Can you work these out from the model? Positions are in its coordinate system, mm. A direction names the side the tool comes from. Round coordinates to 2 decimals unless told otherwise and drop trailing zeros. Order: outer loops, then holes, each group sorted by start corner. A loop starts at its lowest first (then second) coordinate and runs counter-clockwise, first axis right, second up. Notation, with made-up numbers: M 58.25,7.5 L 115.25,7.5 A7 ccw 115.25,19.5 Z; hole C 44,-19 d2. An arc over 180 degrees is marked long. One line per question, with ' | ' between items.
```python
from build123d import *

# Parameters (mm, degrees)
BOSS_EXTRUDE1_DEPTH = 3
SKETCH2_R           = 2
BOSS_EXTRUDE2_DEPTH = 10
SKETCH3_R           = 1.1
CUT_EXTRUDE1_DEPTH  = 10
SKETCH4_W           = 26.4
SKETCH4_H           = 15.8
SKETCH4_W_2         = 22.4
SKETCH4_H_2         = 11.8
BOSS_EXTRUDE3_DEPTH = 4.3
BOSS_EXTRUDE4_DEPTH = 4.3
SKETCH6_R           = 1.1
CUT_EXTRUDE2_DEPTH  = 20.3
SKETCH7_W           = 16.276669309
SKETCH7_H           = 13.12120508
CUT_EXTRUDE3_DEPTH  = 20.3
BOSS_EXTRUDE5_DEPTH = 3
CUT_EXTRUDE4_START  = -21
SKETCH10_R          = 2
CUT_EXTRUDE4_DEPTH  = 21


with BuildPart() as part:
    # Sketch1 → Boss-Extrude1 (new body)
    with BuildSketch(Plane(origin=(0, 0, 0), x_dir=(1, 0, 0), z_dir=(0, 1, 0))):
        with BuildLine():
            Line((-30.38926404, 6.174917902), (-40.065448474, 32.76001614))
            Line((-40.065448474, 32.76001614), (40.065448474, 32.76001614))
            Line((40.065448474, 32.76001614), (30.38926404, 6.174917902))
            ThreePointArc((30.38926404, 6.174917902), (30.206247108, 3.382619115), (31.552193238, 0.929283279))
            Line((31.552193238, 0.929283279), (33.658129878, -1.17665336))
            ThreePointArc((33.658129878, -1.17665336), (34.741993634, -2.798770105), (35.122595972, -4.712187266))
            Line((35.122595972, -4.712187266), (35.122595972, -23.310725409))
            Line((35.122595972, -23.310725409), (-35.122595972, -23.310725409))
            Line((-35.122595972, -23.310725409), (-35.122595972, -4.712187266))
            ThreePointArc((-35.122595972, -4.712187266), (-34.741993634, -2.798770105), (-33.658129878, -1.17665336))
            Line((-33.658129878, -1.17665336), (-31.552193238, 0.929283279))
            ThreePointArc((-31.552193238, 0.929283279), (-30.206247108, 3.382619115), (-30.38926404, 6.174917902))
        make_face()
    extrude(amount=BOSS_EXTRUDE1_DEPTH)

    # Sketch2 → Boss-Extrude2 (add)
    with BuildSketch(Plane(origin=(0, 3, 0), x_dir=(1, 0, 0), z_dir=(0, 1, 0))):
        with Locations(Location((17.5, 0, 0), (0, 0, 270))):
            Circle(SKETCH2_R)
        with Locations(Location((-17.5, 0, 0), (0, 0, 270))):
            Circle(SKETCH2_R)
    extrude(amount=BOSS_EXTRUDE2_DEPTH)

    # Sketch3 → Cut-Extrude1 (cut)
    with BuildSketch(Plane(origin=(0, 3, 0), x_dir=(1, 0, 0), z_dir=(0, 1, 0))):
        with Locations(Location((-31.300794494, -15.24150981, 0), (0, 0, 270))):
            Circle(SKETCH3_R)
        with Locations(Location((-3.502149082, -14.967077195, 0), (0, 0, 270))):
            Circle(SKETCH3_R)
    extrude(amount=-CUT_EXTRUDE1_DEPTH, mode=Mode.SUBTRACT)

    # Sketch4 → Boss-Extrude3 (add)
    with BuildSketch(Plane.XZ):
        with Locations((-17.401471788, 15.214861671)):
            Rectangle(SKETCH4_W, SKETCH4_H)
        with Locations((-17.401471788, 15.214861671)):
            Rectangle(SKETCH4_W_2, SKETCH4_H_2, mode=Mode.SUBTRACT)
    extrude(amount=BOSS_EXTRUDE3_DEPTH)

    # Sketch5 → Boss-Extrude4 (add)
    with BuildSketch(Plane.XZ):
        Polygon((-30.601471788, 23.114861671), (-30.601471788, 7.314861671), (-33.601471788, 9.046912478), (-33.601471788, 21.382810863), align=None)
        Polygon((-1.201471788, 21.382810863), (-4.201471788, 23.114861671), (-4.201471788, 7.314861671), (-1.201471788, 9.046912478), align=None)
    extrude(amount=BOSS_EXTRUDE4_DEPTH)

    # Sketch6 → Cut-Extrude2 (cut)
    with BuildSketch(Plane(origin=(0, 3, 0), x_dir=(1, 0, 0), z_dir=(0, 1, 0))):
        with Locations(Location((-31.300794494, -15.24150981, 0), (0, 0, 270))):
            Circle(SKETCH6_R)
        with Locations(Location((-3.502149082, -14.967077195, 0), (0, 0, 270))):
            Circle(SKETCH6_R)
    extrude(amount=-CUT_EXTRUDE2_DEPTH, mode=Mode.SUBTRACT)

    # Sketch7 → Cut-Extrude3 (cut)
    with BuildSketch(Plane.XZ):
        with Locations((-13.786077898, 14.682620826)):
            Rectangle(SKETCH7_W, SKETCH7_H)
    extrude(amount=-CUT_EXTRUDE3_DEPTH, mode=Mode.SUBTRACT)

    # Sketch8 → Boss-Extrude5 (add)
    with BuildSketch(Plane(origin=(0, 3, 0), x_dir=(1, 0, 0), z_dir=(0, 1, 0))):
        Polygon((-35.122595972, -23.310725409), (35.122595972, -23.310725409), (25.122595972, -33.310725409), (-25.122595972, -33.310725409), align=None)
    extrude(amount=-BOSS_EXTRUDE5_DEPTH)

    # Sketch10 → Cut-Extrude4 (cut)
    with BuildSketch(Plane(origin=(0, 13, 0), x_dir=(1, 0, 0), z_dir=(0, 1, 0)).offset(CUT_EXTRUDE4_START)):
        with Locations(Location((-17.5, 0, 0), (0, 0, 270))):
            Circle(SKETCH10_R)
        with Locations(Location((17.5, 0, 0), (0, 0, 270))):
            Circle(SKETCH10_R)
    extrude(amount=CUT_EXTRUDE4_DEPTH, mode=Mode.SUBTRACT)


solid = part.part
```
(1) If we section it at C-C on x = 17.5: Please give me the cut outline in (y, z).
Final values:
outline: M 0,-32.76 L 3,-32.76 L 3,-2 L 0,-2 Z; M 0,2 L 3,2 L 3,33.31 L 0,33.31 Z
(2) If we section it at A-A on z = 18: Please give me the cut outline in (x, y).
Final values:
outline: M -35.12,0 L -33.6,0 L -33.6,-4.3 L -28.6,-4.3 L -28.6,0 L -21.92,0 L -21.92,3 L -35.12,3 Z; M -6.2,-4.3 L -1.2,-4.3 L -1.2,0 L 35.12,0 L 35.12,3 L -5.65,3 L -5.65,0 L -6.2,0 Z
(3) On a 3-axis mill with a long thin cutter (end or side, diameter ignored), from which of +Z, -Z, +X, -X, +Y, -Y can I reach the whole of each face in a straight line? I mean faces 4 (the flat face through (35.295, 1.479, -19.654)), 5 (the flat face through (-32.12, -2.12, 22.24)), 6 (the flat face through (-32.08, -2.12, 8.17)), 7 (the flat face through (-18, -2, 23.115)). Say none if no direction works.
Final values:
face 4: +X, +Y, -Y | face 5: +Z, -X, -Y | face 6: -Z, -X, -Y | face 7: +Z, +X, -X, -Y
(4) Will these pins go through, and if not, where does the flat tip stop? pin 1 Ø0.9 at (y, z) = (1.5, 18.5) entering from +X; pin 2 Ø1 at (x, z) = (5, 25.5) entering from -Y; pin 3 Ø2 at (y, z) = (1.5, 13) entering from -X.
Final values:
pin 1: x = 35.12 | pin 2: y = 0 | pin 3: x = -35.12
(5) If we section it at B-B on x = -17.5: Please give me the cut outline in (y, z), plus the area to 3 significant figures.
Final values:
outline: M -4.3,7.31 L 0,7.31 L 0,2 L 3,2 L 3,8.12 L 0,8.12 L 0,9.31 L -4.3,9.31 Z; M -4.3,21.11 L 0,21.11 L 0,21.24 L 3,21.24 L 3,33.31 L 0,33.31 L 0,23.11 L -4.3,23.11 Z; M 0,-32.76 L 3,-32.76 L 3,-2 L 0,-2 Z | area: 164 mm^2
(6) If we section it at D-D on z = 0: Please give me the cut outline in (x, y).
Final values:
outline: M -32.48,0 L -19.5,0 L -19.5,3 L -32.48,3 Z; M -15.5,0 L 15.5,0 L 15.5,3 L -15.5,3 Z; M 19.5,0 L 32.48,0 L 32.48,3 L 19.5,3 Z
(7) Please list where these lines run through material, in increasing order: probe 1 along X at (y, z) = (-3.5, 18); probe 2 along Z at (x, y) = (-17.5, 1.25); probe 3 along X at (y, z) = (1.75, 14.5). Write a range as [from, to].
Final values:
probe 1: [-33.6, -28.6], [-6.2, -1.2] | probe 2: [-32.76, -2], [2, 8.12], [21.24, 33.31] | probe 3: [-35.12, -32.11], [-30.49, -21.92], [-5.65, -4.5], [-2.51, 35.12]
(8) Thinking about a two-plate mould opening in Z: for faces 1 (the flat face through (-30.053, 1.521, 28.381)), 2 (the flat face through (-25, 0, 15)), 3 (the flat face through (-18, -2, 7.315)), which applies, released by +Z, released by -Z, zero draft, split by the parting line, or undercut?
Final values:
face 1: released by +Z | face 2: undercut | face 3: released by -Z
